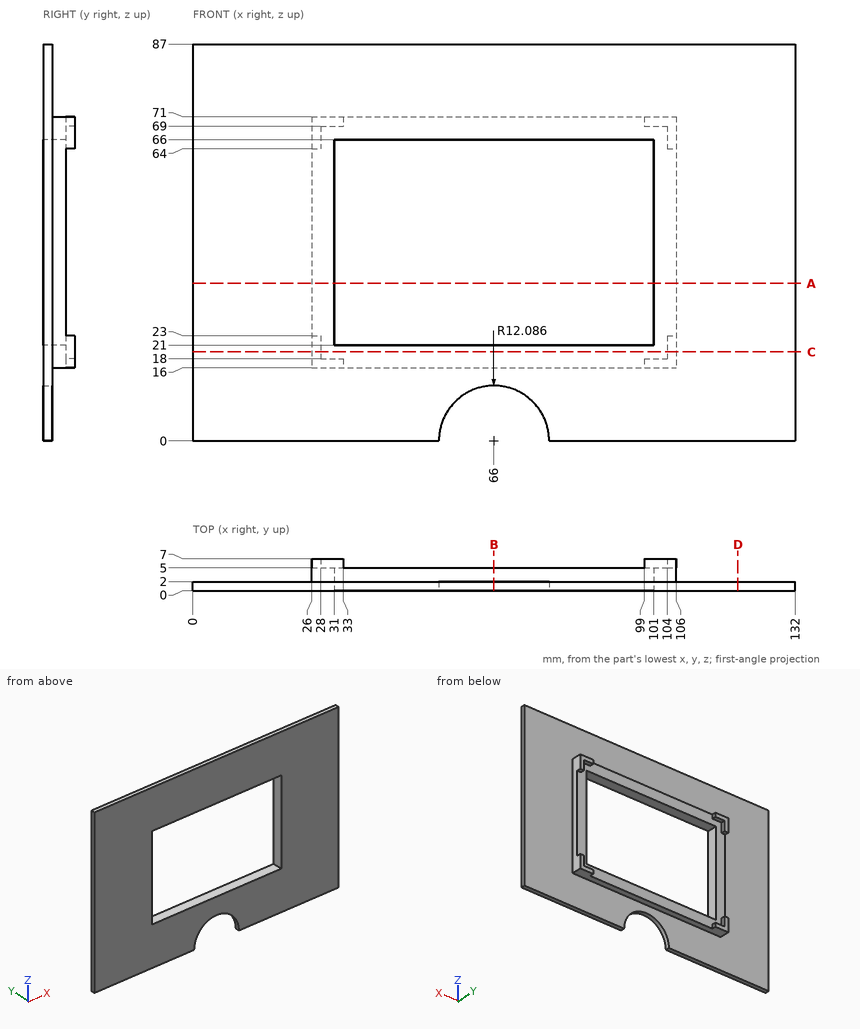
Design review of the part shown in the three views and the two pictorial views. Dimensions are in mm from the part's minimum x, y and z. Round coordinates to 2 decimals unless told otherwise and drop trailing zeros. Order: outer loops, then holes, each group sorted by start corner. A loop starts at its lowest first (then second) coordinate and runs counter-clockwise, first axis right, second up.
Item 1: To check wall thickness, follow probe 1 along X at (y, z) = (4.25, 58); probe 2 along Z at (x, y) = (90, 0.5); probe 3 along Z at (x, y) = (85.5, 3.5). State the ranges of each line that lie inside material, in increasing order.
Working result:
probe 1: x = 26 to 31, 101 to 106
probe 2: z = 0 to 21, 66 to 87
probe 3: z = 16 to 21, 66 to 71
Item 2: Add section D-D, the plane x = 119.5. State the section outline as (y, z) points.
Working result:
outline: (0, 0) - (2, 0) - (2, 87) - (0, 87) - close
Item 3: For pin 1 (1.6 mm diameter, centred on y = 6.5, z = 21, fed in from -X); pin 2 (1 mm diameter, centred on y = 6, z = 69.5, fed in from +X); pin 3 (2 mm diameter, centred on x = 27.5, y = 5.5, fed in from -Z), all flat-tipped, find the tip position at first contact; note any pin that passes through.
Working result:
pin 1: stops at x = 26
pin 2: stops at x = 106
pin 3: stops at z = 16
Item 4: Add section A-A, the plane z = 34.5. State the section outline as (x, y) points, and give its area (3 significant figures).
Working result:
outline: (0, 0) - (31, 0) - (31, 5) - (26, 5) - (26, 2) - (0, 2) - close; (101, 0) - (132, 0) - (132, 2) - (106, 2) - (106, 5) - (101, 5) - close
area: 154 mm2
Item 5: Add section C-C, the plane z = 19.5. State the section outline as (x, y) points, and give its area (3 significant figures).
Working result:
outline: (0, 0) - (132, 0) - (132, 2) - (106, 2) - (106, 7) - (104, 7) - (104, 5) - (28, 5) - (28, 7) - (26, 7) - (26, 2) - (0, 2) - close
area: 512 mm2
Item 6: Add section B-B, the plane x = 66. State the section outline as (y, z) points (1 decimal).
Working result:
outline: (0, 12.1) - (2, 12.1) - (2, 16) - (5, 16) - (5, 21) - (0, 21) - close; (0, 66) - (5, 66) - (5, 71) - (2, 71) - (2, 87) - (0, 87) - close
